Could you check a few things on this model? Use its own coordinates, in mm. A direction names the side the tool comes from. Give positions to 0.01 mm unless a question says otherwise; leave off trailing zeros. Order: outer loops, then holes, each group sorted by start corner. A loop starts at its lowest first (then second) coordinate and runs counter-clockwise, first axis right, second up. Notation, with made-up numbers: M 34,25 L 58,25 A18 ccw 58,40 Z; hole C 72,61.5 d4. An arc over 180 degrees is marked long. Use a Markdown table: item, result. Add a question column.
Item 1: Suppose I cut it at C-C on y = -67. Write out the boundary of the cut face in (x, z), plus the area to 3 significant figures.
Item 2: Suppose I cut it at B-B on x = 0. Count the separate pieces of the cut face and the enclosed holes in it, plus the area to 3 significant figures.
Item 3: Suppose I cut it at D-D on z = -169. Write out the boundary of the cut face in (x, y), plus the area to 3 significant figures.
Item 4: I'm going to push flat-ended pins straight in: pin 1 Ø5 at (x, z) = (-1, -100.5) entering from -Y; pin 2 Ø1.5 at (x, z) = (0, -70.5) entering from -Y. Where does each tip first touch, or does it pass through?
Item 5: Suppose I cut it at A-A on z = -70.5. Write out the boundary of the cut face in (x, y), plus the area to 3 significant figures.
Item 6: For faces 1 (the face through (-2, 0, -86)), 2 (the face through (0.07, -15.8, -346.13)), which set-ups out of +Z, -Z, +X, -X, +Y, -Y let a thin tool reach every point of the face, with its end or its side?
Item 7: If I drill on L1, parallel to Y at x = 0.5, z = -24; L2, parallel to Z at x = 2.25, y = -69; L3, parallel to Z at x = -2.25, y = -72, over which ranges is the centre line in solid material (lowest first)? Write a range as from..to.
Autodesk Inventor part; units mm, degrees
ref_plane "YZ Plane" through (0, 0, 0) normal (1, 0, 0) x (0, 1, 0)
ref_plane "XZ Plane" through (0, 0, 0) normal (0, 1, 0) x (-1, 0, 0)
ref_plane "XY Plane" through (0, 0, 0) normal (0, 0, 1) x (1, 0, 0)
sketch "Sketch1" plane through (0, 0, 0) normal (0, 1, 0) x (-1, 0, 0)
  line L0 (0, 0) -> (0, -180) construction
  line L1 (5, 0) -> (5, -180)
  line L2 (-5, -180) -> (-5, 0)
  arc A0 (5, 0) -> (-5, 0) centre (0, 0) ccw
  arc A1 (-5, -180) -> (5, -180) centre (0, -180) ccw
  circle A2 centre (0, 0) radius 1.65
  line L3 (0, -40) -> (0, -140) construction
  line L4 (1.65, -40) -> (1.65, -140)
  line L5 (-1.65, -140) -> (-1.65, -40)
  arc A3 (1.65, -40) -> (-1.65, -40) centre (0, -40) ccw
  arc A4 (-1.65, -140) -> (1.65, -140) centre (0, -140) ccw
  point P0 (0, -90)
  point P1 (0, -90)
  dimension "d0" = 180
  dimension "d1" = 10
  dimension "d2" = 3.3
  dimension "d3" = 40
  dimension "d5" = 140
  dimension "d6" = 3.3
extrude "Extrusion1" add sketch "Sketch1" along normal blind 6
sketch "Sketch2" plane through (5, 0, 0) normal (1, 0, 0) x (0, 0, -1)
  line L0 (180, 0) -> (180, 6)
  line L1 (0, 0) -> (180, 0)
  line L2 (180, 0) -> (180, 6)
  line L3 (0, 6) -> (180, 6)
  line L4 (0, 0) -> (0, 6)
  line L5 (180, 0) -> (180, 0)
  line L6 (180, 0) -> (180, 6)
  line L7 (180, 6) -> (180, 6)
  line L8 (180, 0) -> (180, 6)
  line L9 (180, 0) -> (0, 0)
  arc A0 (498.004, -84) -> (180, 0) centre (180, -643.9437) ccw
  line L10 (180, 6) -> (0, 6)
  arc A1 (498.004, -78) -> (180, 6) centre (180, -637.9437) ccw
  line L11 (498.004, -78) -> (498.004, -84)
  line L12 (0, 0) -> (180, 0)
  dimension "d9" = 6
  dimension "d10" = 498.004
  dimension "d11" = 90
extrude "Extrusion2" add sketch "Sketch2" against normal blind 10 contours L0 A1 L11 A0
fillet "Fillet1" radius 2 4 edges at (0, -78, -498.004) (5, -81, -498.004) (-5, -81, -498.004) (0, -84, -498.004)
Findings below:
| question | item | result |
|---|---|---|
| 1 | outline | M -5,-477.8 L 5,-477.8 L 5,-466.01 L -5,-466.01 Z |
| 1 | area | 118 mm^2 |
| 2 | separate pieces | 3 |
| 2 | enclosed holes | 0 |
| 2 | area | 2,380 mm^2 |
| 3 | outline | M -5,0 L 5,0 L 5,6 L -5,6 Z |
| 3 | area | 60.0 mm^2 |
| 4 | pin 1 | stops at y = 0 |
| 4 | pin 2 | passes through |
| 5 | outline | M -5,0 L -1.65,0 L -1.65,6 L -5,6 Z; M 1.65,0 L 5,0 L 5,6 L 1.65,6 Z |
| 5 | area | 40.2 mm^2 |
| 6 | face 1 | +Z, +X, -X, -Y |
| 6 | face 2 | -Z, +X, -X, +Y |
| 7 | L1 | y = 0..6 |
| 7 | L2 | z = -481.61..-470.01 |
| 7 | L3 | z = -487.2..-475.88 |
